Model file for the job. Use its own axes, mm. A direction names the side the tool comes from. Coordinates: 2 decimals unless noted, no trailing zeros. Order: outer loops, then holes, each group sorted by start corner. A loop starts at its lowest first (then second) coordinate and runs counter-clockwise, first axis right, second up.
from build123d import *

# Parameters (mm, degrees)
F0_W             = 1
F0_H             = 20
F1_DEPTH         = 19
F2_W             = 50
F2_H             = 18.5
F3_DEPTH         = 17.2
F4_W             = 46
F4_H             = 18.5
F5_DEPTH         = 0.5
F7_DEPTH         = 11
F10_DEPTH        = 5
F8_R             = 7
F11_DEPTH        = 15
F12_R            = 1.25
F13_DEPTH        = 4
F13_COPIES_COUNT = 8


# Not quite as in the source:
# - a pattern or mirror of a feature is missing from the dataset's text; its kind, count and spacing are read off the source's solid


with BuildPart() as f1:
    # F0 (on Top) → F1 (new body)
    with BuildSketch(Plane.XY):
        with BuildLine():
            ThreePointArc((-36.0123676672, -10), (5.0462056754, -37.0327751226), (37.375, 0))
            ThreePointArc((37.375, 0), (5.0462056754, 37.0327751226), (-36.0123676672, 10))
            Line((-36.0123676672, 10), (-30, 10))
            Line((-30, 10), (-30, -10))
            Line((-30, -10), (-36.0123676672, -10))
        make_face()
        with BuildLine():
            Line((-30, 10), (-36.0123676672, 10))
            ThreePointArc((-36.0123676672, 10), (-37.375, 0), (-36.0123676672, -10))
            Line((-36.0123676672, -10), (-30, -10))
            Line((-30, -10), (-30, 10))
        make_face()
        with BuildLine():
            ThreePointArc((-36.0123676672, -10), (-37.375, 0), (-36.0123676672, 10))
            Line((-36.0123676672, 10), (-44.75, 10))
            Line((-44.75, 10), (-44.75, -10))
            Line((-44.75, -10), (-36.0123676672, -10))
        make_face()
        with Locations((-45.25, 0)):
            Rectangle(F0_W, F0_H)
    extrude(amount=F1_DEPTH)

    # F2 (on face) → F3 (cut)
    with BuildSketch(Plane(origin=(0, 0, 0), x_dir=(1, 0, 0), z_dir=(0, 0, -1))):
        with Locations((-20.75, 0)):
            Rectangle(F2_W, F2_H)
    extrude(amount=-F3_DEPTH, mode=Mode.SUBTRACT)

    # F4 (on face) → F5 (cut)
    with BuildSketch(Plane(origin=(0, 0, 17.2), x_dir=(1, 0, 0), z_dir=(0, 0, -1))):
        with Locations((-20.75, 0)):
            Rectangle(F4_W, F4_H)
    extrude(amount=-F5_DEPTH, mode=Mode.SUBTRACT)

    # F6 (on face) → F7 (cut)
    with BuildSketch(Plane(origin=(0, 0, 0), x_dir=(1, 0, 0), z_dir=(0, 0, -1))):
        Polygon((30.5, 20.4567786688), (4.25, 20.4567786688), (4.25, 9.25), (4.25, -9.25), (4.25, -19.5432213312), (30.5, -19.5432213312), align=None)
    extrude(amount=-F7_DEPTH, mode=Mode.SUBTRACT)

    # F9 (on face) → F10 (cut)
    with BuildSketch(Plane(origin=(0, 0, 0), x_dir=(1, 0, 0), z_dir=(0, 0, -1))):
        Polygon((-27.0342712475, -9.25), (-12.8921356237, -23.3921356237), (1.25, -9.25), align=None)
    extrude(amount=-F10_DEPTH, mode=Mode.SUBTRACT)

    # F8 (on face) → F11 (cut)
    with BuildSketch(Plane(origin=(0, 0, 0), x_dir=(1, 0, 0), z_dir=(0, 0, -1))):
        with Locations((-12.8315193579, -23.0468716472)):
            Circle(F8_R)
    extrude(amount=-F11_DEPTH, mode=Mode.SUBTRACT)

    # F12 (on face) → F13 (cut)
    with BuildSketch(Plane(origin=(0, 0, 15), x_dir=(1, 0, 0), z_dir=(0, 0, -1))):
        with Locations((-12.8591003243, -17.7969360865)):
            Circle(F12_R)
    f13 = extrude(amount=-F13_DEPTH, mode=Mode.SUBTRACT)

    # F13_copies: F13 ×8 about axis
    f13_copies_axis = Axis((-12.831519, 23.046872, 0), (0, 0, 1))
    for i in range(1, F13_COPIES_COUNT):
        add(f13.rotate(f13_copies_axis, i * 360 / F13_COPIES_COUNT), mode=Mode.SUBTRACT)


solid = f1.part
Q1. Probe line 1 (Z direction, x = -11.5, y = 2); line 2 (Z direction, x = 5.5, y = -19.5); line 3 (Y direction, x = -17.5, z = 13.75). List the from-to ranges inside material, lowest first.
Established:
line 1: z = 17.7 to 19
line 2: z = 11 to 19
line 3: y = -33.02 to -9.25, 9.25 to 17.83, 28.26 to 33.02
Q2. Cut at D-D, the plane y = 13. List the corners of the cut face in (x, z).
Established:
outline: (-35.04, 0) - (-23.28, 0) - (-23.28, 5) - (-2.5, 5) - (-2.5, 0) - (4.25, 0) - (4.25, 11) - (30.5, 11) - (30.5, 0) - (35.04, 0) - (35.04, 19) - (-35.04, 19) - close
Q3. Drop flat-ended pins along their axis: P1, Ø3, axis at x = -16.56, y = 19.35, coming from the -Z side; P2, Ø8, axis at y = 21.5, z = 15, coming from the -X side; P3, Ø8, axis at x = -43, z = 6.5, coming from the -Y side. Give the stop position or say it passes through.
Established:
P1: stops at z = 15
P2: stops at x = -33.02
P3: stops at y = -10
Q4. Cut at A-A, the plane x = 0. List the corners of the cut face in (y, z) (3 decimals).
Established:
outline: (-37.375, 0) - (-9.25, 0) - (-9.25, 17.7) - (9.25, 17.7) - (9.25, 5) - (10.5, 5) - (10.5, 0) - (37.375, 0) - (37.375, 19) - (-37.375, 19) - close
Q5. Cut at B-B, the plane z = 14. List the corners of the cut face in (x, y) (3 decimals).
Established:
outline: (-45.75, -10) - (-36.012, -10) arc R37.375 ccw (long way) to (-36.012, 10) - (-45.75, 10) - (-45.75, 9.25) - (4.25, 9.25) - (4.25, -9.25) - (-45.75, -9.25) - close; hole circle Ø14 at (-12.832, 23.047)
Q6. Mould opens along X. For faces 1 (the face through (-3.3, 13.8, 2.5)), 2 (the face through (-41, 10, 9)) say: pulls with the +X half, pulls with the -X half, needs draft (parallel to the pull), parting line crosses it, or undercut.
Established:
face 1: undercut
face 2: needs draft
Q7. Cut at C-C, the plane y = 0. List the corners of the cut face in (x, z) (3 decimals), plus the area to 3 significant figures.
Established:
outline: (-45.75, 17.2) - (-43.75, 17.2) - (-43.75, 17.7) - (2.25, 17.7) - (2.25, 17.2) - (4.25, 17.2) - (4.25, 11) - (30.5, 11) - (30.5, 0) - (37.375, 0) - (37.375, 19) - (-45.75, 19) - close
area: 408 mm2
Q8. Which spindle directions (+Z, -Z, +X, -X, +Y, -Y) get a long thin tool onto all of the face, cutting with end or side? Do faces 3 (the face through (3, 0, 17.2)), 4 (the face through (4.25, -15, 5)), 5 (the face through (-41, -10, 9)), 6 (the face through (-5, -16, 0)), 7 (the face through (-15.68, 27.7, 16.97)). Say none if no direction does.
Established:
face 3: -Z, -X
face 4: -Z
face 5: +Z, -Z, -X, -Y
face 6: -Z, +X, -X, +Y, -Y
face 7: +Z, -Z
